Source: CAD feature listing. Evaluate the final solid. Frame: model axes, mm. Give positions to 0.01 mm unless a question says otherwise; leave off trailing zeros. Write each loop counter-clockwise with the first axis right and the second up, starting at its lowest first coordinate (ties: lowest second). Pieces come first, ordered by that corner, then holes.
```python
from build123d import *

# Parameters (mm, degrees)
SKIZZE1_W                       = 180
SKIZZE1_H                       = 110
AUFSATZ_LINEAR_AUSTRAGEN1_DEPTH = 15
SKIZZE2_R                       = 2.75
SCHNITT_LINEAR_AUSTRAGEN1_DEPTH = 40
SKIZZE3_R                       = 3
SCHNITT_LINEAR_AUSTRAGEN2_DEPTH = 40


with BuildPart() as part:
    # Skizze1 → Aufsatz-Linear austragen1 (new body)
    with BuildSketch(Plane.XY):
        with Locations((0, 55)):
            Rectangle(SKIZZE1_W, SKIZZE1_H)
    extrude(amount=AUFSATZ_LINEAR_AUSTRAGEN1_DEPTH)

    # Skizze2 → Schnitt-Linear austragen1 (cut)
    with BuildSketch(Plane.XY.offset(15)):
        with Locations((34, 24)):
            Circle(SKIZZE2_R)
        with Locations((70, 24)):
            Circle(SKIZZE2_R)
        with Locations(Location((70, 56, 0), (0, 0, 180))):
            Circle(SKIZZE2_R)
        with Locations(Location((34, 56, 0), (0, 0, 180))):
            Circle(SKIZZE2_R)
        with Locations(Location((-34, 24, 0), (0, 0, 180))):
            Circle(SKIZZE2_R)
        with Locations(Location((-70, 24, 0), (0, 0, 180))):
            Circle(SKIZZE2_R)
        with Locations((-70, 56)):
            Circle(SKIZZE2_R)
        with Locations((-34, 56)):
            Circle(SKIZZE2_R)
    extrude(amount=-SCHNITT_LINEAR_AUSTRAGEN1_DEPTH, mode=Mode.SUBTRACT)

    # Skizze3 → Schnitt-Linear austragen2 (cut)
    with BuildSketch(Plane.XY.offset(15)):
        with Locations((52, 85)):
            Circle(SKIZZE3_R)
        with Locations(Location((-52, 85, 0), (0, 0, 180))):
            Circle(SKIZZE3_R)
    extrude(amount=-SCHNITT_LINEAR_AUSTRAGEN2_DEPTH, mode=Mode.SUBTRACT)


solid = part.part
```
1. Cut plane B-B, the plane y = 56. Return the cut outline in (x, z).
2. Line query: L1, parallel to Y at x = 34, z = 4.25; L2, parallel to Y at x = -72, z = 9; L3, parallel to Y at x = 52, z = 6.75. Output: solid intervals per line, ascending.
3. Cut plane C-C, the plane x = 70. Return the cut outline in (y, z), then the cut area to 4 significant figures.
4. Mould query, pull axis Y, two halves, no side actions, for faces 1 (the cylindrical face through (-51.35, 87.93, 7.6)), 2 (the flat face through (-1, 56, 15)), 3 (the flat face through (-1, 110, 7)). Classes: +Y half, -Y half, draft (parallel to the pull), parting line (faces both ways), or undercut.
5. Contact query for flat-ended pins moving along their axis: P1, Ø9, axis at x = -70, y = 24, coming from the +Z side; P2, Ø3.5, axis at x = 52, y = 85, coming from the +Z side. Output: stop coordinate, or through.
6. Cut plane A-A, the plane x = -52. Return the cut outline in (y, z).
Response values:
1. outline: (-90, 0) - (-72.75, 0) - (-72.75, 15) - (-90, 15) - close; (-67.25, 0) - (-36.75, 0) - (-36.75, 15) - (-67.25, 15) - close; (-31.25, 0) - (31.25, 0) - (31.25, 15) - (-31.25, 15) - close; (36.75, 0) - (67.25, 0) - (67.25, 15) - (36.75, 15) - close; (72.75, 0) - (90, 0) - (90, 15) - (72.75, 15) - close
2. L1: y = 0 to 21.25, 26.75 to 53.25, 58.75 to 110
2. L2: y = 0 to 22.11, 25.89 to 54.11, 57.89 to 110
2. L3: y = 0 to 82, 88 to 110
3. outline: (0, 0) - (21.25, 0) - (21.25, 15) - (0, 15) - close; (26.75, 0) - (53.25, 0) - (53.25, 15) - (26.75, 15) - close; (58.75, 0) - (110, 0) - (110, 15) - (58.75, 15) - close
3. area: 1,485 mm2
4. face 1: undercut
4. face 2: draft
4. face 3: +Y half
5. P1: stops at z = 15
5. P2: passes through
6. outline: (0, 0) - (82, 0) - (82, 15) - (0, 15) - close; (88, 0) - (110, 0) - (110, 15) - (88, 15) - close
